Can you work these out from the model? Positions are in its coordinate system, mm. Face numbers are marked on the shaded views. A direction names the side the tool comes from. Give positions to 0.01 mm unless a question says otherwise; leave off trailing zeros. Write each loop counter-clockwise with the first axis right and the second up, starting at its lowest first coordinate (ties: lowest second). Pieces come first, ordered by that corner, then holes.
from build123d import *

# Parameters (mm, degrees)
SKETCH_1_W          = 90
SKETCH_1_H          = 80
SKETCH_1_R          = 1.5
EXTRUDE_1_DEPTH     = 1.5
SKETCH_2_W          = 13
SKETCH_2_H          = 8
EXTRUDE_2_DEPTH     = 4
SKETCH_3_W          = 13
SKETCH_3_H          = 8
SKETCH_3_W_2        = 10
SKETCH_3_H_2        = 12
EXTRUDE_3_DEPTH     = 15
SKETCH_4_R          = 1.762202075
SKETCH_4_R_2        = 1.721763756
CUT_EXTRUDE_1_DEPTH = 4


with BuildPart() as part:
    # Sketch 1 → Extrude 1 (new body)
    with BuildSketch(Plane.XY):
        with Locations((45, 40)):
            Rectangle(SKETCH_1_W, SKETCH_1_H)
        with Locations((4, 76)):
            Circle(SKETCH_1_R, mode=Mode.SUBTRACT)
        with Locations(Location((86, 76, 0), (0, 0, 180))):
            Circle(SKETCH_1_R, mode=Mode.SUBTRACT)
        with Locations((86, 4)):
            Circle(SKETCH_1_R, mode=Mode.SUBTRACT)
        with Locations(Location((4, 4, 0), (0, 0, 180))):
            Circle(SKETCH_1_R, mode=Mode.SUBTRACT)
    extrude(amount=EXTRUDE_1_DEPTH)



with BuildPart() as body_2:
    # Sketch 2 → Extrude 2 (new body)
    with BuildSketch(Plane.XZ):
        with Locations((29.5, -4)):
            Rectangle(SKETCH_2_W, SKETCH_2_H)
    extrude(amount=EXTRUDE_2_DEPTH)


with BuildPart() as part_1:
    add(part.part)

    add(body_2.part)  # Extrude 3 merges body 2
    # Sketch 3 → Extrude 3 (add)
    with BuildSketch(Plane(origin=(0, 0, 0), x_dir=(1, 0, 0), z_dir=(0, 1, 0))):
        with Locations((29.5, 4)):
            Rectangle(SKETCH_3_W, SKETCH_3_H)
        with Locations((15, 6)):
            Rectangle(SKETCH_3_W_2, SKETCH_3_H_2)
    extrude(amount=EXTRUDE_3_DEPTH)

    # Sketch 4 → Cut-Extrude 1 (cut)
    with BuildSketch(Plane.XZ.offset(4)):
        Polygon((25.156072285, -1.21963674), (23.853575099, -2.522133926), (23.853575099, -5.586833186), (25.002837322, -6.736095409), (35.116344883, -6.736095409), (35.116344883, -1.21963674), align=None)
        with Locations(Location((26.611804434, -3.977866074, 0), (0, 0, 270))):
            Circle(SKETCH_4_R, mode=Mode.SUBTRACT)
        with Locations(Location((32.43473303, -3.977866074, 0), (0, 0, 270))):
            Circle(SKETCH_4_R_2, mode=Mode.SUBTRACT)
    extrude(amount=-CUT_EXTRUDE_1_DEPTH, mode=Mode.SUBTRACT)


solid = part_1.part
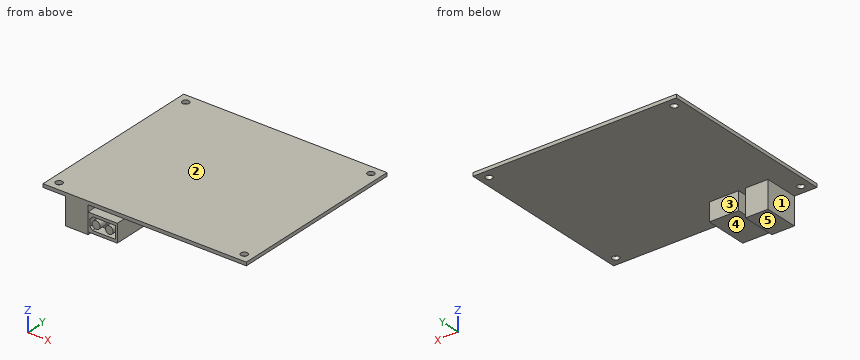
(1) Imagine slicing it at A-A, the plane x = 4. Write out the boundary of the cut face in (y, z), plus the area to 3 significant figures.
Returned:
outline: (0, 0) - (2.5, 0) - (2.5, 1.5) - (0, 1.5) - close; (5.5, 0) - (74.5, 0) - (74.5, 1.5) - (5.5, 1.5) - close; (77.5, 0) - (80, 0) - (80, 1.5) - (77.5, 1.5) - close
area: 111 mm2
(2) Imagine slicing it at C-C, the plane y = 4. Write out the boundary of the cut face in (x, z), plus the area to 3 significant figures.
Returned:
outline: (0, 0) - (2.5, 0) - (2.5, 1.5) - (0, 1.5) - close; (5.5, 0) - (10, 0) - (10, -12) - (20, -12) - (20, 0) - (23, 0) - (23, -8) - (36, -8) - (36, 0) - (84.5, 0) - (84.5, 1.5) - (5.5, 1.5) - close; (87.5, 0) - (90, 0) - (90, 1.5) - (87.5, 1.5) - close
area: 350 mm2
(3) For the marked faces 1, 2, 3, 4 and 5, which set-ups out of +Z, -Z, +X, -X, +Y, -Y let a thin tool reach every point of the face, with its end or its side?
Returned:
face 1: -Z, -X, +Y, -Y
face 2: +Z, +X, -X, +Y, -Y
face 3: -Z, +X, -X, +Y
face 4: -Z, +X, +Y, -Y
face 5: -Z, +X, -X, +Y, -Y
(4) If I drill on L1, parallel to Y at x = 86, z = 1.2; L2, parallel to X at y = 76, z = 0.95; L3, parallel to Z at x = 23, y = 55, over which ranges is the centre line in solid material (lowest first)?
Returned:
L1: y = 0 to 2.5, 5.5 to 74.5, 77.5 to 80
L2: x = 0 to 2.5, 5.5 to 84.5, 87.5 to 90
L3: z = 0 to 1.5
(5) Imagine slicing it at D-D, the plane x = 71.5. Write out the boundary of the cut face in (y, z).
Returned:
outline: (0, 0) - (80, 0) - (80, 1.5) - (0, 1.5) - close
(6) Will these pins go through, and if not, where does the flat tip stop? P1, Ø3.5, axis at y = 6, z = -4.5, coming from the -X side; P2, Ø10.5, axis at x = 30.5, y = 7.5, coming from the -Z side; P3, Ø3.5, axis at x = 86, y = 4, coming from the +Z side; P4, Ø1.2, axis at x = 31, y = -2, coming from the +Z side.
Returned:
P1: stops at x = 10
P2: stops at z = -8
P3: stops at z = 1.5
P4: stops at z = 0
(7) Imagine slicing it at B-B, the plane y = 76. Write out the boundary of the cut face in (x, z), plus the area to 3 significant figures.
Returned:
outline: (0, 0) - (2.5, 0) - (2.5, 1.5) - (0, 1.5) - close; (5.5, 0) - (84.5, 0) - (84.5, 1.5) - (5.5, 1.5) - close; (87.5, 0) - (90, 0) - (90, 1.5) - (87.5, 1.5) - close
area: 126 mm2
